Autodesk Inventor part; units mm, degrees
ref_plane "YZ Plane" through (0, 0, 0) normal (1, 0, 0) x (0, 1, 0)
ref_plane "XZ Plane" through (0, 0, 0) normal (0, 1, 0) x (-1, 0, 0)
ref_plane "XY Plane" through (0, 0, 0) normal (0, 0, 1) x (1, 0, 0)
ref_plane "Work Plane1" through (29.0854, -74.8946, 2) normal (0, 0, 1) x (1, 0, 0)
sketch "Sketch1" plane through (29.0854, -74.8946, 2) normal (0, 0, 1) x (1, 0, 0)
  line L0 (19.0856, -32.3111) -> (19.0856, -42.3111)
  line L1 (29.0856, -32.3111) -> (19.0856, -32.3111)
  line L2 (29.0856, -42.3111) -> (29.0856, -32.3111)
  line L3 (19.0856, -42.3111) -> (29.0856, -42.3111)
  circle A0 centre (32.6545, -45.7111) radius 1.45
  point P0 (-29.0854, 74.8946)
  dimension "d1" = 2.9
extrude "Extrusion1" add sketch "Sketch1" along normal blind 17.9 contours A0
sketch "Sketch2" plane through (61.7399, -120.6057, 19.9) normal (0, 0, 1) x (1, 0, 0)
  circle A0 centre (0, 0) radius 1.45
  circle A1 centre (0, 0) radius 2.915
  point P0 (-61.7399, 120.6057)
  dimension "d4" = 5.83
extrude "Extrusion2" add sketch "Sketch2" along normal blind 1.35 contours A0 | A1
ref_plane "Work Plane2" through (61.7399, -120.6057, 22.26) normal (0, 0, 1) x (1, 0, 0)
sketch "Sketch3" plane through (61.7399, -120.6057, 22.26) normal (0, 0, 1) x (1, 0, 0)
  circle A0 centre (0, 0) radius 1.45 construction
  circle A1 centre (0, 0) radius 1.1446
  point P0 (-61.7399, 120.6057)
loft "Loft1" add profiles "Sketch3" section 1 edges at (58.8249, -120.6057, 21.25)
ref_plane "Work Plane3" through (61.7399, -120.6057, 19.9) normal (0, 0, -1) x (-1, 0, 0)
properties part number "screw"
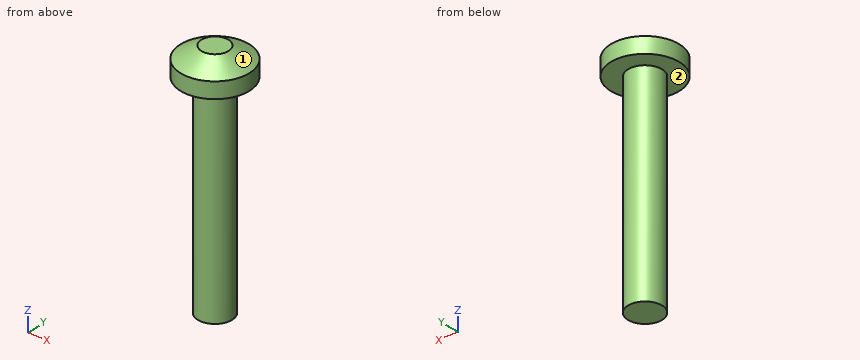
Here's how the part is built. I have some questions about the finished solid (model axes, mm). Face numbers are marked on the shaded views. A direction names the side the tool comes from. Give positions to 0.01 mm unless a question says otherwise; leave off trailing zeros. Loops run counter-clockwise (first coordinate to the right, second up) from the corner with the lowest first, then second, coordinate; pieces in that order, holes last. Notation, with made-up numbers: (15.5, -21) -> (26.5, -21) arc R20 ccw to (26.5, 14) -> close; hole circle Ø4 at (19.5, 37). An arc over 180 degrees is marked (long way). Use one line per item in the form item = value. Start each with the question number.
1) Please list where these lines run through material, in increasing order: line 1 along X through (y, z) = (-120.6, 18); line 2 along X through (y, z) = (-119.5, 5.75); line 3 along Z through (x, y) = (63.05, -120.45).
2) Imagine slicing it at B-B (z = 20.25). Please give me the cut outline in (x, y) (3 decimals).
3) Imagine slicing it at A-A (z = 6.25). Please give me the cut outline in (x, y).
4) For P1, Ø2, axis at x = 59.5, y = -119.5, coming from the +Z side; P2, Ø1, axis at y = -120, z = 13.5, coming from the -X side; P3, Ø3, axis at x = 63, z = 13.5, coming from the +Y side, each with a flat end and sliding along its axis, tell me the tip position at first contact or that it passes through.
5) Which directions (+Z, -Z, +X, -X, +Y, -Y) give clear straight access to the entire face, cutting with the end or side of a thin tool? Please do the marked faces 1 and 2.
Check values:
q1.line_1 = 60.29 to 63.19
q1.line_2 = 60.8 to 62.68
q1.line_3 = 2 to 22.16
q2.outline = circle Ø5.83 at (61.74, -120.606)
q3.outline = circle Ø2.9 at (61.74, -120.61)
q4.P1 = 22.06
q4.P2 = 60.29
q4.P3 = -119.16
q5.face_1 = +Z
q5.face_2 = -Z
